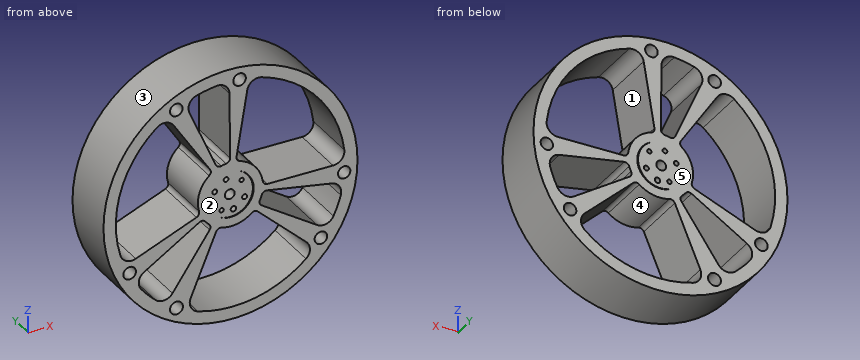
```python
from build123d import *

# Parameters (mm, degrees)
F0_R     = 55.507491
F0_R_2   = 2.831016
F0_R_3   = 2.762544
F0_R_4   = 2.741928
F0_R_5   = 2.700224
F0_R_6   = 2.762824
F0_R_7   = 10.141613
F0_R_8   = 2.750086
F1_DEPTH = 25
F2_R     = 10.141613
F2_R_2   = 0.972579
F2_R_3   = 1.194025
F2_R_4   = 1.098643
F2_R_5   = 1.068939
F2_R_6   = 1.045628
F2_R_7   = 2.154273
F2_R_8   = 0.934876
F3_DEPTH = 25


with BuildPart() as f1:
    # F0 (on Front) → F1 (new body)
    with BuildSketch(Plane.XZ):
        Circle(F0_R)
        with Locations((-23.60731, -43.971572)):
            Circle(F0_R_2, mode=Mode.SUBTRACT)
        with Locations((-44.092819, -22.890553)):
            Circle(F0_R_3, mode=Mode.SUBTRACT)
        with BuildLine():
            ThreePointArc((-38.981074, -31.501106), (-40.027301, -27.555651), (-37.784517, -24.145208))
            Line((-37.784517, -24.145208), (-13.582291, -8.679408))
            ThreePointArc((-13.582291, -8.679408), (-12.196485, -8.388691), (-10.965496, -9.088434))
            ThreePointArc((-10.965496, -9.088434), (-10.231273, -9.907714), (-9.436002, -10.667877))
            ThreePointArc((-9.436002, -10.667877), (-8.776165, -11.92071), (-9.11125, -13.296461))
            Line((-9.11125, -13.296461), (-25.346547, -36.989368))
            ThreePointArc((-25.346547, -36.989368), (-28.827279, -39.121436), (-32.737088, -37.949003))
            ThreePointArc((-32.737088, -37.949003), (-36.003715, -34.865115), (-38.981074, -31.501106))
        make_face(mode=Mode.SUBTRACT)
        with BuildLine():
            ThreePointArc((9.250821, -10.828853), (10.583292, -10.349798), (11.89902, -10.87309))
            Line((11.89902, -10.87309), (33.101832, -30.247802))
            ThreePointArc((33.101832, -30.247802), (34.728727, -33.991385), (33.023564, -37.699973))
            ThreePointArc((33.023564, -37.699973), (10.726868, -48.9569), (-14.234037, -48.05451))
            ThreePointArc((-14.234037, -48.05451), (-17.333693, -45.398699), (-17.421203, -41.317823))
            Line((-17.421203, -41.317823), (-6.262349, -14.852398))
            ThreePointArc((-6.262349, -14.852398), (-5.285977, -13.826888), (-3.875272, -13.70489))
            ThreePointArc((-3.875272, -13.70489), (3.048283, -13.912214), (9.250821, -10.828853))
        make_face(mode=Mode.SUBTRACT)
        with Locations((39.516639, -30.155763)):
            Circle(F0_R_4, mode=Mode.SUBTRACT)
        with BuildLine():
            ThreePointArc((45.023811, -22.015908), (41.89017, -24.631533), (37.851417, -24.040197))
            Line((37.851417, -24.040197), (13.606339, -8.64166))
            ThreePointArc((13.606339, -8.64166), (12.757193, -7.508556), (12.871137, -6.097177))
            ThreePointArc((12.871137, -6.097177), (13.303361, -5.085501), (13.656207, -4.043482))
            ThreePointArc((13.656207, -4.043482), (14.512799, -2.915997), (15.901267, -2.63827))
            Line((15.901267, -2.63827), (44.235666, -7.339391))
            ThreePointArc((44.235666, -7.339391), (47.638996, -9.592954), (48.228768, -13.631936))
            ThreePointArc((48.228768, -13.631936), (46.814353, -17.895813), (45.023811, -22.015908))
        make_face(mode=Mode.SUBTRACT)
        with Locations((49.685858, -3.912825)):
            Circle(F0_R_5, mode=Mode.SUBTRACT)
        with BuildLine():
            ThreePointArc((-8.91513, 13.428746), (-8.600271, 12.048225), (-9.278424, 10.805211))
            ThreePointArc((-9.278424, 10.805211), (-13.625701, 4.145118), (-13.723839, -3.80762))
            ThreePointArc((-13.723839, -3.80762), (-13.852795, -5.217706), (-14.883109, -6.189008))
            Line((-14.883109, -6.189008), (-41.403257, -17.217175))
            ThreePointArc((-41.403257, -17.217175), (-45.483651, -17.109536), (-48.124141, -13.996816))
            ThreePointArc((-48.124141, -13.996816), (-47.948665, 14.586616), (-32.176622, 38.425366))
            ThreePointArc((-32.176622, 38.425366), (-28.250027, 39.540292), (-24.800961, 37.357371))
            Line((-24.800961, 37.357371), (-8.91513, 13.428746))
        make_face(mode=Mode.SUBTRACT)
        with BuildLine():
            ThreePointArc((-14.834567, 47.872533), (-10.488232, 49.008578), (-6.057631, 49.750868))
            ThreePointArc((-6.057631, 49.750868), (-2.15728, 48.547347), (-0.453554, 44.838099))
            Line((-0.453554, 44.838099), (-0.163038, 16.117821))
            ThreePointArc((-0.163038, 16.117821), (-0.650861, 14.788535), (-1.896601, 14.115404))
            ThreePointArc((-1.896601, 14.115404), (-2.980469, 13.9269), (-4.046554, 13.655297))
            ThreePointArc((-4.046554, 13.655297), (-5.458676, 13.759623), (-6.447811, 14.772829))
            Line((-6.447811, 14.772829), (-17.937139, 41.09647))
            ThreePointArc((-17.937139, 41.09647), (-17.900729, 45.178121), (-14.834567, 47.872533))
        make_face(mode=Mode.SUBTRACT)
        with Locations((-23.679955, 43.914214)):
            Circle(F0_R_6, mode=Mode.SUBTRACT)
        Circle(F0_R_7, mode=Mode.SUBTRACT)
        with BuildLine():
            Line((2.63827, 15.901267), (7.339391, 44.235666))
            ThreePointArc((7.339391, 44.235666), (9.592954, 47.638996), (13.631936, 48.228768))
            ThreePointArc((13.631936, 48.228768), (38.065025, 32.602111), (49.750868, 6.057631))
            ThreePointArc((49.750868, 6.057631), (48.547347, 2.15728), (44.838099, 0.453554))
            Line((44.838099, 0.453554), (16.117821, 0.163038))
            ThreePointArc((16.117821, 0.163038), (14.788535, 0.650861), (14.115404, 1.896601))
            ThreePointArc((14.115404, 1.896601), (10.817041, 9.26463), (4.043482, 13.656207))
            ThreePointArc((4.043482, 13.656207), (2.915997, 14.512799), (2.63827, 15.901267))
        make_face(mode=Mode.SUBTRACT)
        with Locations((3.962071, 49.823198)):
            Circle(F0_R_8, mode=Mode.SUBTRACT)
    extrude(amount=F1_DEPTH)

    # F2 (on Front) → F3 (join)
    with BuildSketch(Plane.XZ):
        with Locations((-0.332667, 0.152715)):
            Circle(F2_R)
        with Locations((-3.896208, -6.036293)):
            Circle(F2_R_2, mode=Mode.SUBTRACT)
        with Locations((1.296153, -6.800671)):
            Circle(F2_R_3, mode=Mode.SUBTRACT)
        with Locations((6.186505, -2.763281)):
            Circle(F2_R_4, mode=Mode.SUBTRACT)
        with Locations((-6.896846, 2.965934)):
            Circle(F2_R_5, mode=Mode.SUBTRACT)
        with Locations((-1.922125, 7.090822)):
            Circle(F2_R_6, mode=Mode.SUBTRACT)
        with Locations((-0.332667, 0.152715)):
            Circle(F2_R_7, mode=Mode.SUBTRACT)
        with Locations((4.879461, 5.034964)):
            Circle(F2_R_8, mode=Mode.SUBTRACT)
    extrude(amount=F3_DEPTH)


solid = f1.part
```
Design review of the part built by this model. Coordinates are the model's own, in mm. Face numbers are marked on the shaded views. A direction names the side the tool comes from. Give positions to 0.01 mm unless a question says otherwise; leave off trailing zeros. Write each loop counter-clockwise with the first axis right and the second up, starting at its lowest first coordinate (ties: lowest second). Pieces come first, ordered by that corner, then holes. Notation, with made-up numbers: (-31.5, -11.5) -> (17.5, -11.5) arc R26 cw to (17.5, 5.5) -> close; hole circle Ø4 at (-39.5, 35). An arc over 180 degrees is marked (long way). Answer in a Markdown table with one row per item.
(1) Consider section B-B (y = -3.5). Count the separate pieces of the cut face and the enclosed holes in it, then the cut area to 3 significant figures.
Results:
| item | result |
|---|---|
| separate pieces | 1 |
| enclosed holes | 20 |
| area | 3,560 mm2 |
(2) Consider section A-A (x = 18). State the section outline as (y, z) points, then the cut area to 3 significant figures.
Results:
| item | result |
|---|---|
| outline | (-25, -52.51) -> (0, -52.51) -> (0, -46.77) -> (-25, -46.77) -> close; (-25, -16.45) -> (0, -16.45) -> (0, -11.43) -> (-25, -11.43) -> close; (-25, -2.99) -> (0, -2.99) -> (0, 0.18) -> (-25, 0.18) -> close; (-25, 46.77) -> (0, 46.77) -> (0, 52.51) -> (-25, 52.51) -> close |
| area | 491 mm2 |
(3) Clearance check with flat-ended pins moving along their axes: pin 1 (1.9 mm diameter, centred on x = -1.92, z = 7.09, fed in from +Y); pin 2 (3 mm diameter, centred on x = -2.5, y = -4, fed in from -Z); pin 3 (3 mm diameter, centred on y = -19, z = 15.5, fed in from -X); pin 4 (3 mm diameter, centred on x = 10.5, y = -19, fed in from -Z). State where each tip first meets the part, or that it passes through.
Results:
| item | result |
|---|---|
| pin 1 | through |
| pin 2 | z = -55.5 |
| pin 3 | x = -53.71 |
| pin 4 | z = -54.77 |
(4) To check wall thickness, follow probe 1 along Z at (x, y) = (-6, -9); probe 2 along Z at (x, y) = (-38.5, -6.25); probe 3 along Z at (x, y) = (37.5, -13). State the ranges of each line that lie inside material, in increasing order.
Results:
| item | result |
|---|---|
| probe 1 | -55.18 to -49.76, -14.4 to 2.38, 3.55 to 14.13, 49.76 to 55.18 |
| probe 2 | -39.99 to -32.09, -24.7 to -16.01, 32.09 to 39.99 |
| probe 3 | -40.92 to -32.01, -28.3 to -23.82, -6.22 to 0.38, 33.25 to 40.92 |
(5) For the marked faces 1 and 2, list the 3-axis set-ups (+Z, -Z, +X, -X, +Y, -Y) from which the entire face can be reached by the end or side of a thin tool; tool diameter is ignored.
Results:
| item | result |
|---|---|
| face 1 | +Y, -Y |
| face 2 | +Z, -Z, +X, -X, -Y |
(6) Mouldability with a two-part tool opening along X and no side actions: class the marked faces 3, 4 and 5 as +X half, -X half, draft (parallel to the pull), parting line (faces both ways), or undercut.
Results:
| item | result |
|---|---|
| face 3 | parting line |
| face 4 | undercut |
| face 5 | draft |
